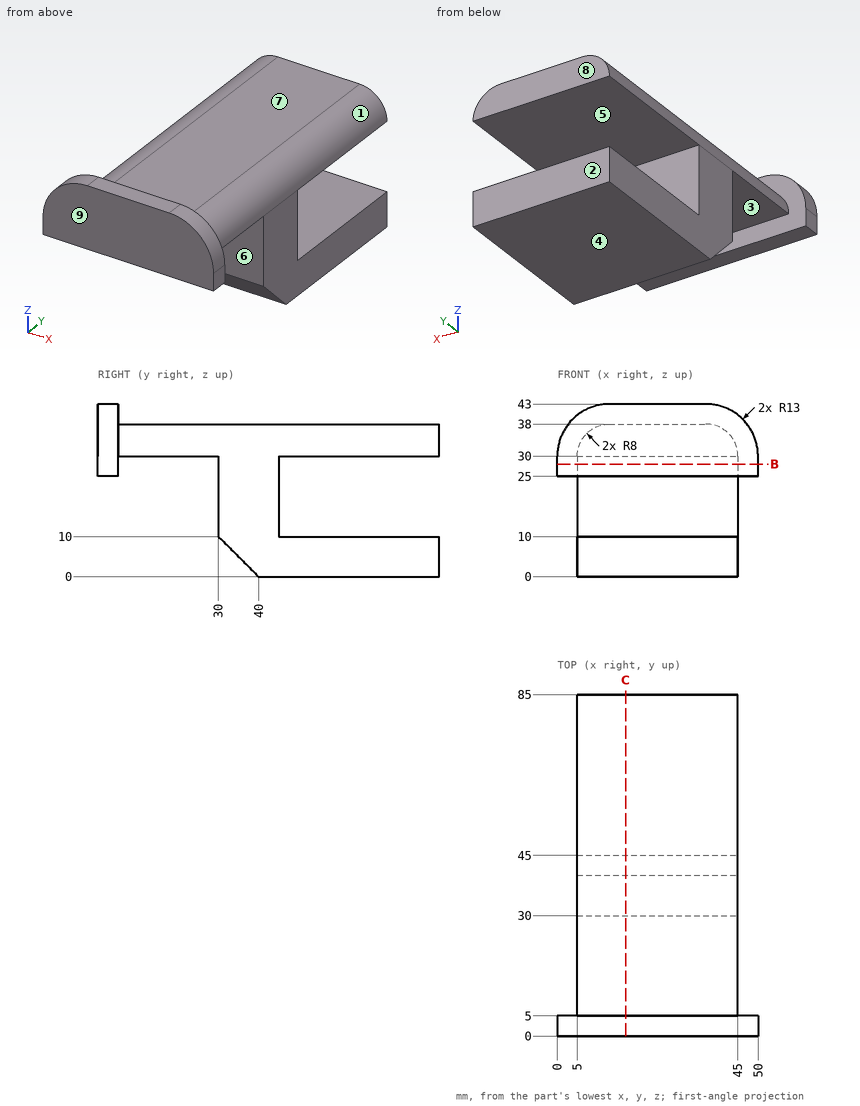
Source: three-view drawing plus pictorial views. Frame: mm from the lowest corner of the part. A direction names the side the tool comes from. Coordinates: 2 decimals unless noted, no trailing zeros. Loops run counter-clockwise (first coordinate to the right, second up) from the corner with the lowest first, then second, coordinate; pieces in that order, holes last. Notation, with made-up numbers: (64, 24) -> (99, 24) arc R32 cw to (99, 54) -> close; hole circle Ø7 at (-12.5, -8.75). An arc over 180 degrees is marked (long way). Write each question's results on one line, items separated by ' | '. Start each with the question number.
Q1. Section C-C, the plane x = 17. Return the cut outline in (y, z), plus the area to 3 significant figures.
Q2. Pin query (flat end, axial travel): pin 1 (3 mm diameter, centred on y = 45.5, z = 17.5, fed in from -X); pin 2 (12 mm diameter, centred on x = 34, y = 21, fed in from -Z); pin 3 (20 mm diameter, centred on x = 20.5, y = 69, fed in from +Z). Return the tip coordinate at first contact, or that it passes through.
Q3. Pull-direction query (Y, two-part tool) for the marked faces 6, 7, 8 and 9; classes: released by +Y, released by -Y, zero draft, split by the parting line, or undercut.
Q4. Section B-B, the plane z = 28. Return the cut outline in (x, y).
Q5. Ray query, line 1 (Z direction, x = 33, y = 71); line 2 (Y direction, x = 20, z = 26.5); line 3 (X direction, y = 45.5, z = 7.5). Return the intervals inside material, ascending. Write a range as from..to.
Q6. Reachability of the marked faces 1, 2, 3, 4 and 5 from +Z, -Z, +X, -X, +Y, -Y: full face, straight path, thin tool, end or side. Return the list, or none.
Found:
1) outline: (0, 25) -> (5, 25) -> (5, 30) -> (30, 30) -> (30, 10) -> (40, 0) -> (85, 0) -> (85, 10) -> (45, 10) -> (45, 30) -> (85, 30) -> (85, 38) -> (5, 38) -> (5, 43) -> (0, 43) -> close | area: 1,530 mm2
2) pin 1: x = 5 | pin 2: z = 30 | pin 3: z = 38
3) face 6: undercut | face 7: zero draft | face 8: released by +Y | face 9: released by -Y
4) outline: (0, 0) -> (50, 0) -> (50, 5) -> (0, 5) -> close; (5, 30) -> (45, 30) -> (45, 45) -> (5, 45) -> close
5) line 1: 0..10, 30..38 | line 2: 0..5, 30..45 | line 3: 5..45
6) face 1: +Z, +X, +Y | face 2: +Z, -Z, +X, -X, +Y | face 3: -Z, +X, -X | face 4: -Z, +X, -X, +Y, -Y | face 5: +X, -X, +Y
